```python
from build123d import *

# Parameters (mm, degrees)
RESSALTO_EXTRUS_O1_DEPTH = 57.75
ESBO_O2_R                = 37.5
RESSALTO_EXTRUS_O2_DEPTH = 1
CORTE_EXTRUS_O1_DEPTH    = 336.452306595
CASCA1_START             = -47.75
CASCA1_OUTLINE_R         = 22.75
CASCA1_DEPTH             = 95.5
CASCA1_START_2           = 281
CASCA1_2_OUTLINE_R       = 27.5
CASCA1_2_DEPTH           = 1
CORTE_EXTRUS_O2_REACH    = 389.923
ESBO_O6_R                = 6
CORTE_EXTRUS_O3_REACH    = 337.452
CORTE_EXTRUS_O4_DEPTH    = 5
ESBO_O9_R                = 2
CORTE_EXTRUS_O5_DEPTH    = 5


with BuildPart() as part:
    # Esboço1 → Ressalto-extrusão1 (new, symmetric)
    with BuildSketch(Plane.XY):
        with BuildLine():
            Line((291, 0), (291, 17))
            Line((291, 17), (274, 17))
            Line((274, 17), (57, 45.607017004))
            ThreePointArc((57, 45.607017004), (-48.32227677, 54.71706834), (-52.304922539, -50.92342367))
            Line((-52.304922539, -50.92342367), (13, -118))
            Line((13, -118), (191, -118))
            Line((191, -118), (291, -101))
            Line((291, -101), (291, 0))
        make_face()
    extrude(amount=RESSALTO_EXTRUS_O1_DEPTH, both=True)

    # Esboço2 → Ressalto-extrusão2 (add, symmetric)
    with BuildSketch(Plane(origin=(291, 0, 0), x_dir=(0, 0, -1), z_dir=(1, 0, 0))):
        with Locations(Location((0.25, -42, 0), (0, 0, 180))):
            Circle(ESBO_O2_R)
    extrude(amount=RESSALTO_EXTRUS_O2_DEPTH, both=True)

    # Esboço4 → Corte-extrusão1 (cut, through all)
    with BuildSketch(Plane(origin=(0, 0, -57.75), x_dir=(-1, 0, 0), z_dir=(0, 0, -1))):
        with BuildLine():
            Line((-2.35, 9.3), (2.35, 9.3))
            Line((2.35, 9.3), (2.35, 12.531560158))
            ThreePointArc((2.35, 12.531560158), (9.01561146, 9.01561146), (12.531560158, 2.35))
            Line((12.531560158, 2.35), (9.3, 2.35))
            Line((9.3, 2.35), (9.3, -2.35))
            Line((9.3, -2.35), (12.531560158, -2.35))
            ThreePointArc((12.531560158, -2.35), (9.01561146, -9.01561146), (2.35, -12.531560158))
            Line((2.35, -12.531560158), (2.35, -9.3))
            Line((2.35, -9.3), (-2.35, -9.3))
            Line((-2.35, -9.3), (-2.35, -12.531560158))
            ThreePointArc((-2.35, -12.531560158), (-9.01561146, -9.01561146), (-12.531560158, -2.35))
            Line((-12.531560158, -2.35), (-9.3, -2.35))
            Line((-9.3, -2.35), (-9.3, 2.35))
            Line((-9.3, 2.35), (-12.531560158, 2.35))
            ThreePointArc((-12.531560158, 2.35), (-9.01561146, 9.01561146), (-2.35, 12.531560158))
            Line((-2.35, 12.531560158), (-2.35, 9.3))
        make_face()
    extrude(amount=-CORTE_EXTRUS_O1_DEPTH, mode=Mode.SUBTRACT)

    # Casca1: read off the stored shape, not the designer's step
    # Casca1 outline → Casca1 (cut)
    with BuildSketch(Plane.XY.offset(CASCA1_START)):
        with BuildLine():
            ThreePointArc((51.532195013, 36.241314506), (-40.221654164, 48.489365187), (-45.139864657, -43.947612208))
            Line((-45.139864657, -43.947612208), (17.22074544, -108))
            Line((17.22074544, -108), (190.15605408, -108))
            Line((190.15605408, -108), (281, -92.556529194))
            Line((281, -92.556529194), (281, 7))
            Line((281, 7), (273.343691363, 7))
            Line((273.343691363, 7), (51.532195013, 36.241314506))
        make_face()
        Circle(CASCA1_OUTLINE_R, mode=Mode.SUBTRACT)
    extrude(amount=CASCA1_DEPTH, mode=Mode.SUBTRACT)

    # Casca1 2 outline → Casca1 2 (cut)
    with BuildSketch(Plane.YZ.offset(CASCA1_START_2)):
        with Locations((-42, -0.25)):
            Circle(CASCA1_2_OUTLINE_R)
    extrude(amount=CASCA1_2_DEPTH, mode=Mode.SUBTRACT)

    # Esboço6 → Corte-extrusão2 (cut, up to next)
    with BuildSketch(Plane(origin=(292, 0, 0), x_dir=(0, 0, -1), z_dir=(1, 0, 0)), mode=Mode.PRIVATE) as corte_extrus_o2_sk1:
        with Locations((0.25, -42)):
            Circle(ESBO_O6_R)
    corte_extrus_o2_tool1 = extrude(corte_extrus_o2_sk1.sketch, amount=-CORTE_EXTRUS_O2_REACH, mode=Mode.PRIVATE) & part.part
    add(corte_extrus_o2_tool1.solids().sort_by_distance((292, -42, -0.25))[0], mode=Mode.SUBTRACT)

    # Esboço7 → Corte-extrusão3 (cut, up to next)
    with BuildSketch(Plane.XY.offset(57.75), mode=Mode.PRIVATE) as corte_extrus_o3_sk1:
        with BuildLine():
            Line((245, -88), (115, -88))
            ThreePointArc((115, -88), (107.928932188, -85.071067812), (105, -78))
            Line((105, -78), (105, -18))
            ThreePointArc((105, -18), (107.928932188, -10.928932188), (115, -8))
            Line((115, -8), (245, -8))
            ThreePointArc((245, -8), (252.071067812, -10.928932188), (255, -18))
            Line((255, -18), (255, -78))
            ThreePointArc((255, -78), (252.071067812, -85.071067812), (245, -88))
        make_face()
    corte_extrus_o3_tool1 = extrude(corte_extrus_o3_sk1.sketch, amount=-CORTE_EXTRUS_O3_REACH, mode=Mode.PRIVATE) & part.part
    add(corte_extrus_o3_tool1.solids().sort_by_distance((180, -48, 57.75))[0], mode=Mode.SUBTRACT)

    # Esboço8 → Corte-extrusão4 (cut)
    with BuildSketch(Plane.XY.offset(57.75)):
        with BuildLine():
            Line((255, -98), (105, -98))
            ThreePointArc((105, -98), (97.928932188, -95.071067812), (95, -88))
            Line((95, -88), (95, -8))
            ThreePointArc((95, -8), (97.928932188, -0.928932188), (105, 2))
            Line((105, 2), (255, 2))
            ThreePointArc((255, 2), (262.071067812, -0.928932188), (265, -8))
            Line((265, -8), (265, -88))
            ThreePointArc((265, -88), (262.071067812, -95.071067812), (255, -98))
        make_face()
    extrude(amount=-CORTE_EXTRUS_O4_DEPTH, mode=Mode.SUBTRACT)

    # Esboço9 → Corte-extrusão5 (cut)
    with BuildSketch(Plane.XY.offset(52.75)):
        with Locations((180, -3)):
            Circle(ESBO_O9_R)
        with Locations((260, -48)):
            Circle(ESBO_O9_R)
        with Locations((180, -93)):
            Circle(ESBO_O9_R)
        with Locations((99.997152321, -48)):
            Circle(ESBO_O9_R)
    extrude(amount=-CORTE_EXTRUS_O5_DEPTH, mode=Mode.SUBTRACT)


solid = part.part
```
Build history of the part. All positions in model axes, mm. A direction names the side the tool comes from. Coordinates: 2 decimals unless noted, no trailing zeros. Order: outer loops, then holes, each group sorted by start corner. A loop starts at its lowest first (then second) coordinate and runs counter-clockwise, first axis right, second up. Notation, with made-up numbers: (25, 80.25) -> (56, 80.25) arc R19 cw to (56, 91.25) -> close; hole circle Ø6 at (81, -34). An arc over 180 degrees is marked (long way). Answer in a Markdown table with one row per item. Add a question column.
Q1. Wall check: line 1 along X through (y, z) = (1.5, 12.5); line 2 along Z through (x, y) = (11.5, -79); line 3 along Z through (x, y) = (175, -88.5). Give the ranges that are in metal, low to high. Write a range as [from, to].
Q2. Band-saw the part on D-D, the plane x = 161. List the corners of the cut face in (y, z), then the cut area to 3 significant figures.
Q3. Mould opens along Y. For faces 1 (the face through (240.3, -109.62, 0.81)), 2 (the face through (66, -21, 57.75)), 3 (the face through (180, -7, 52.75)) say: +Y half, -Y half, draft (parallel to the pull), parting line (faces both ways), or undercut.
Q4. Band-saw the part on B-B, the plane x = 86.5. List the corners of the cut face in (y, z), then the cut area to 3 significant figures.
Q5. Band-saw the part on C-C, the plane z = -16. Give the number of separate pieces and of enclosed holes in the cut face, then the cut area to 3 significant figures.
Q6. Drop flat-ended pins along their axis: pin 1 (1.4 mm diameter, centred on y = 0, z = -8.5, fed in from -X); pin 2 (3 mm diameter, centred on y = -83.5, z = 18.5, fed in from +X); pin 3 (12 mm diameter, centred on x = -12, z = 13.5, fed in from +Y). Give the stop position or say it passes through.
Q7. Which spindle directions (+Z, -Z, +X, -X, +Y, -Y) get a long thin tool onto all of the face, cutting with end or side? Do faces 4 (the face through (283, 17, 1)), 5 (the face through (251.99, -10.85, 50.28)), 6 (the face through (-14.396, -75.525, -0.669)), 7 (the face through (-20.1, -84, 0.8)). Say none if no direction does.
Q8. Band-saw the part on A-A, the plane y = 50. List the corners of the cut face in (x, z).
Answers follow:
| question | item | result |
|---|---|---|
| 1 | line 1 | [-72.98, -62.98], [-22.7, -9.3], [9.3, 22.7], [281, 291] |
| 1 | line 2 | [-57.75, -47.75], [47.75, 57.75] |
| 1 | line 3 | [-57.75, -47.75], [47.75, 52.75] |
| 2 | outline | (-118, -57.75) -> (31.9, -57.75) -> (31.9, 57.75) -> (2, 57.75) -> (2, 52.75) -> (-8, 52.75) -> (-8, 47.75) -> (21.81, 47.75) -> (21.81, -47.75) -> (-108, -47.75) -> (-108, 47.75) -> (-88, 47.75) -> (-88, 52.75) -> (-98, 52.75) -> (-98, 57.75) -> (-118, 57.75) -> close |
| 2 | area | 4,020 mm^2 |
| 3 | face 1 | -Y half |
| 3 | face 2 | draft |
| 3 | face 3 | undercut |
| 4 | outline | (-118, -57.75) -> (41.72, -57.75) -> (41.72, 57.75) -> (-118, 57.75) -> close; hole (-108, -47.75) -> (31.63, -47.75) -> (31.63, 47.75) -> (-108, 47.75) -> close |
| 4 | area | 5,110 mm^2 |
| 5 | separate pieces | 2 |
| 5 | enclosed holes | 2 |
| 5 | area | 10,500 mm^2 |
| 6 | pin 1 | x = -73 |
| 6 | pin 2 | x = 291 |
| 6 | pin 3 | y = 72.75 |
| 7 | face 4 | +Z, -Z, +X, +Y |
| 7 | face 5 | +Z |
| 7 | face 6 | none |
| 7 | face 7 | +Z, -Z, -X, -Y |
| 8 | outline | (-53.19, -57.75) -> (53.19, -57.75) -> (53.19, 57.75) -> (-53.19, 57.75) -> close; hole (-38.33, -47.75) -> (38.33, -47.75) -> (38.33, 47.75) -> (-38.33, 47.75) -> close |
